```python
from build123d import *

# Parameters (mm, degrees)
SKETCH_1_W          = 48.4
SKETCH_1_H          = 40
SKETCH_1_W_2        = 42.4
SKETCH_1_H_2        = 34
EXTRUDE_1_DEPTH     = 160
SKETCH_2_R          = 2.5
CUT_EXTRUDE_1_DEPTH = 18
CUT_EXTRUDE_START   = -10
SKETCH_4_R          = 2.5
CUT_EXTRUDE_3_DEPTH = 10
SKETCH_8_R          = 1.5
CUT_EXTRUDE_6_DEPTH = 50
CUT_EXTRUDE_7_DEPTH = 10
FILLET_1_R          = 3
CUT_EXTRUDE_8_DEPTH = 10
FILLET_2_R          = 3


with BuildPart() as part:
    # 草图1 → 凸台-拉伸1 (new body)
    with BuildSketch(Plane.XY):
        Rectangle(SKETCH_1_W, SKETCH_1_H)
        Rectangle(SKETCH_1_W_2, SKETCH_1_H_2, mode=Mode.SUBTRACT)
    extrude(amount=EXTRUDE_1_DEPTH)

    # 草图2 → 切除-拉伸1 (cut)
    with BuildSketch(Plane(origin=(24.2, 0, 0), x_dir=(0, 0, -1), z_dir=(1, 0, 0))):
        with Locations((-135, 12)):
            Circle(SKETCH_2_R)
        with Locations((-135, -12)):
            Circle(SKETCH_2_R)
        with Locations((-25, 12)):
            Circle(SKETCH_2_R)
        with Locations((-25, -12)):
            Circle(SKETCH_2_R)
    extrude(amount=-CUT_EXTRUDE_1_DEPTH, mode=Mode.SUBTRACT)

    # 草图4 → 切除-拉伸3 (cut)
    with BuildSketch(Plane.ZY.offset(24.2).offset(CUT_EXTRUDE_START)):
        with Locations(Location((25, 12, 0), (0, 0, 180))):
            Circle(SKETCH_4_R)
        with Locations(Location((25, -12, 0), (0, 0, 180))):
            Circle(SKETCH_4_R)
        with Locations(Location((135, 12, 0), (0, 0, 180))):
            Circle(SKETCH_4_R)
        with Locations(Location((135, -12, 0), (0, 0, 180))):
            Circle(SKETCH_4_R)
    extrude(amount=CUT_EXTRUDE_3_DEPTH, mode=Mode.SUBTRACT)

    # 草图8 → 切除-拉伸6 (cut)
    with BuildSketch(Plane(origin=(0, 20, 0), x_dir=(1, 0, 0), z_dir=(0, 1, 0))):
        with Locations(Location((-15, -44, 0), (0, 0, 180))):
            Circle(SKETCH_8_R)
        with Locations(Location((15, -44, 0), (0, 0, 180))):
            Circle(SKETCH_8_R)
        with Locations(Location((-15, -116, 0), (0, 0, 180))):
            Circle(SKETCH_8_R)
        with Locations(Location((15, -116, 0), (0, 0, 180))):
            Circle(SKETCH_8_R)
    extrude(amount=-CUT_EXTRUDE_6_DEPTH, mode=Mode.SUBTRACT)

    # 草图9 → 切除-拉伸7 (cut)
    with BuildSketch(Plane.XZ.offset(20)):
        Polygon((-21.2, 160), (-14.2, 130), (14.2, 130), (21.2, 160), align=None)
        Polygon((21.2, 0), (-21.2, 0), (-14.2, 30), (14.2, 30), align=None)
    extrude(amount=-CUT_EXTRUDE_7_DEPTH, mode=Mode.SUBTRACT)

    # 圆角1
    fillet_1_edges = [part.edges().sort_by_distance(p)[0] for p in [
        (14.2, -18.5, 130),
        (-14.2, -18.5, 130),
        (-14.2, -18.5, 30),
        (14.2, -18.5, 30),
    ]]
    fillet(fillet_1_edges, radius=FILLET_1_R)

    # 草图10 → 切除-拉伸8 (cut)
    with BuildSketch(Plane(origin=(0, 20, 0), x_dir=(1, 0, 0), z_dir=(0, 1, 0))):
        Polygon((-21.2, 0), (-14.2, -10), (14.2, -10), (21.2, 0), align=None)
        Polygon((21.2, -160), (-21.2, -160), (-14.2, -150), (14.2, -150), align=None)
    extrude(amount=-CUT_EXTRUDE_8_DEPTH, mode=Mode.SUBTRACT)

    # 圆角2
    fillet_2_edges = [part.edges().sort_by_distance(p)[0] for p in [
        (14.2, 18.5, 10),
        (-14.2, 18.5, 10),
        (14.2, 18.5, 150),
        (-14.2, 18.5, 150),
    ]]
    fillet(fillet_2_edges, radius=FILLET_2_R)


solid = part.part
```
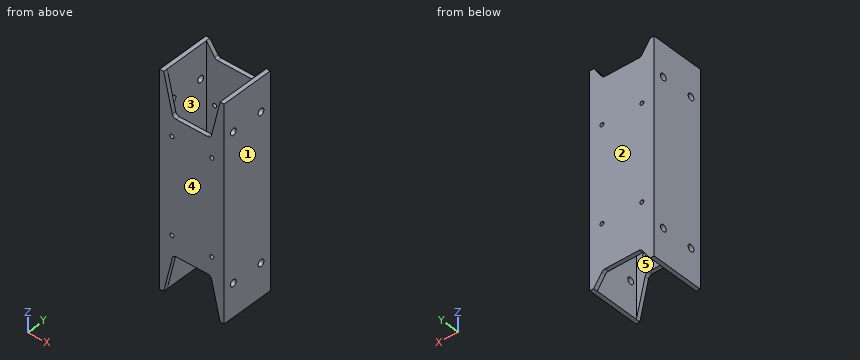
CAD build for the part. Positions are in the model's coordinates, mm. Face numbers are marked on the shaded views. A direction names the side the tool comes from. Give positions to 0.01 mm unless a question says otherwise; leave off trailing zeros. Order: outer loops, then holes, each group sorted by start corner. A loop starts at its lowest first (then second) coordinate and runs counter-clockwise, first axis right, second up.
(1) Drill centre lines: L1, parallel to Z at x = -23.2, y = 12; L2, parallel to X at y = -10.5, z = 100.5; L3, parallel to Y at x = -19, z = 136.5. Where is each one in solid material? Low to high.
(2) Saw through at A-A, the plane z = 116. Give the cut face in (x, y).
(3) Flat gauge pins, fed straight in: pin 1 (0.9 mm diameter, centred on x = 0, y = 19, fed in from -Z); pin 2 (1.5 mm diameter, centred on x = -5, y = -18, fed in from +Z); pin 3 (2.5 mm diameter, centred on x = -5.5, y = 18.5, fed in from +Z). Where does each tip first touch, or does it go through?
(4) Saw through at B-B, the plane y = -1. Give the cut face in (x, z), then the cut area to 3 significant figures.
(5) Mould opens along Y. For the marked faces 1, 2 and 3 say: released by +Y, released by -Y, zero draft, split by the parting line, or undercut.
(6) Saw through at D-D, the plane y = -12. Give the cut face in (x, z).
(7) Tool access for the marked faces 4 and 5: list every direction of +Z, -Z, +X, -X, +Y, -Y with a clear straight run to the whole face (end or side of a thin tool).
(8) Saw through at C-C, the plane x = 5. Give the cut face in (y, z), then the cut area to 3 significant figures.
Results found:
1. L1: z = 0 to 22.5, 27.5 to 132.5, 137.5 to 160
1. L2: x = -24.2 to -21.2, 21.2 to 24.2
1. L3: y = -20 to -17, 17 to 20
2. outline: (-24.2, -20) - (-16.5, -20) - (-16.5, -17) - (-21.2, -17) - (-21.2, 17) - (-16.5, 17) - (-16.5, 20) - (-24.2, 20) - close; (-13.5, -20) - (13.5, -20) - (13.5, -17) - (-13.5, -17) - close; (-13.5, 17) - (13.5, 17) - (13.5, 20) - (-13.5, 20) - close; (16.5, -20) - (24.2, -20) - (24.2, 20) - (16.5, 20) - (16.5, 17) - (21.2, 17) - (21.2, -17) - (16.5, -17) - close
3. pin 1: stops at z = 10
3. pin 2: stops at z = 130
3. pin 3: stops at z = 150
4. outline: (-24.2, 0) - (-21.2, 0) - (-21.2, 160) - (-24.2, 160) - close; (21.2, 0) - (24.2, 0) - (24.2, 160) - (21.2, 160) - close
4. area: 960 mm2
5. face 1: zero draft
5. face 2: released by +Y
5. face 3: undercut
6. outline: (-24.2, 0) - (-21.2, 0) - (-21.2, 22.5) - (-24.2, 22.5) - close; (-24.2, 27.5) - (-21.2, 27.5) - (-21.2, 132.5) - (-24.2, 132.5) - close; (-24.2, 137.5) - (-21.2, 137.5) - (-21.2, 160) - (-24.2, 160) - close; (21.2, 0) - (24.2, 0) - (24.2, 22.5) - (21.2, 22.5) - close; (21.2, 27.5) - (24.2, 27.5) - (24.2, 132.5) - (21.2, 132.5) - close; (21.2, 137.5) - (24.2, 137.5) - (24.2, 160) - (21.2, 160) - close
7. face 4: +Z, -Z, +X, -X, -Y
7. face 5: +Z, -Z
8. outline: (-20, 30) - (-17, 30) - (-17, 130) - (-20, 130) - close; (17, 10) - (20, 10) - (20, 150) - (17, 150) - close
8. area: 720 mm2
